Geometry check sheet. Reference: the model listing, model coordinates, mm. Give positions to 0.01 mm unless a question says otherwise; leave off trailing zeros. Order: outer loops, then holes, each group sorted by start corner. A loop starts at its lowest first (then second) coordinate and runs counter-clockwise, first axis right, second up.
from build123d import *

# Parameters (mm, degrees)
F0_R     = 10
F0_R_2   = 2.5
F1_DEPTH = 20
F2_DEPTH = 25


with BuildPart() as f1:
    # F0 (on Top) → F1 (new body)
    with BuildSketch(Plane.XY):
        with BuildLine():
            ThreePointArc((8.333333, -23.570226), (20.412415, -14.433757), (25, 0))
            ThreePointArc((25, 0), (20.412415, 14.433757), (8.333333, 23.570226))
            ThreePointArc((8.333333, 23.570226), (-25, 0), (8.333333, -23.570226))
        make_face()
        Circle(F0_R, mode=Mode.SUBTRACT)
        with BuildLine():
            ThreePointArc((8.333333, 23.570226), (20.412415, 14.433757), (25, 0))
            ThreePointArc((25, 0), (20.412415, -14.433757), (8.333333, -23.570226))
            Line((8.333333, -23.570226), (61.666667, -4.714045))
            ThreePointArc((61.666667, -4.714045), (55, 0), (61.666667, 4.714045))
            Line((61.666667, 4.714045), (8.333333, 23.570226))
        make_face()
        with BuildLine():
            ThreePointArc((65, 0), (64.082483, 2.886751), (61.666667, 4.714045))
            ThreePointArc((61.666667, 4.714045), (55, 0), (61.666667, -4.714045))
            ThreePointArc((61.666667, -4.714045), (64.082483, -2.886751), (65, 0))
        make_face()
        with Locations((60, 0)):
            Circle(F0_R_2, mode=Mode.SUBTRACT)
    extrude(amount=F1_DEPTH)

    # F0 (on Top) → F2 (join)
    with BuildSketch(Plane.XY):
        with BuildLine():
            ThreePointArc((8.333333, -23.570226), (20.412415, -14.433757), (25, 0))
            ThreePointArc((25, 0), (20.412415, 14.433757), (8.333333, 23.570226))
            ThreePointArc((8.333333, 23.570226), (-25, 0), (8.333333, -23.570226))
        make_face()
        Circle(F0_R, mode=Mode.SUBTRACT)
    extrude(amount=F2_DEPTH)


solid = f1.part
Item 1: Draft check along Y on faces 1 (the flat face through (0, -11, 25)), 2 (the cylindrical face through (62.31, -0.96, 9.86)), 3 (the flat face through (34.627, -14.274, 9.86)). Enter one of: released by +Y, released by -Y, zero draft, split by the parting line, or undercut.
Reported:
face 1: zero draft
face 2: undercut
face 3: released by -Y
Item 2: Sectioned sample at D-D (x = 60). Enter the section's corners in (y, z).
Reported:
outline: (-5.3, 0) - (-2.5, 0) - (-2.5, 20) - (-5.3, 20) - close; (2.5, 0) - (5.3, 0) - (5.3, 20) - (2.5, 20) - close
Item 3: Sectioned sample at B-B (x = 0). Enter the section's corners in (y, z), and give its area (3 significant figures).
Reported:
outline: (-25, 0) - (-10, 0) - (-10, 25) - (-25, 25) - close; (10, 0) - (25, 0) - (25, 25) - (10, 25) - close
area: 750 mm2
Item 4: Sectioned sample at A-A (z = 2.25). Enter the section's corners in (x, y), and give its area (3 significant figures).
Reported:
outline: (8.33, -23.57) - (61.67, -4.71) arc R5 ccw to (61.67, 4.71) - (8.33, 23.57) arc R25 ccw (long way) to start; hole circle Ø20 at (0, 0); hole circle Ø5 at (60, 0)
area: 2,590 mm2
Item 5: Sectioned sample at C-C (y = 9). Enter the section's corners in (x, z), and give its area (3 significant figures).
Reported:
outline: (-23.32, 0) - (-4.36, 0) - (-4.36, 25) - (-23.32, 25) - close; (4.36, 0) - (49.54, 0) - (49.54, 20) - (23.32, 20) - (23.32, 25) - (4.36, 25) - close
area: 1,470 mm2
Item 6: Gauge pin test, flat ends, axial feed: pin 1 (1 mm diameter, centred on y = 1.5, z = 7.5, fed in from +X); pin 2 (6 mm diameter, centred on x = -6.5, z = 17.5, fed in from +Y); pin 3 (10 mm diameter, centred on x = 14, z = 18, fed in from -Y). Record the tip position at first contact, or that the pin passes through.
Reported:
pin 1: stops at x = 64.9
pin 2: stops at y = 24.75
pin 3: stops at y = -23.33
Item 7: Scan lines: L1, parallel to Y at x = 0, z = 19.5; L2, parallel to Y at x = 60, z = 14.75; L3, parallel to X at y = 3.5, z = 14.5. Record each from-to range of solid material in increasing order.
Reported:
L1: y = -25 to -10, 10 to 25
L2: y = -5.3 to -2.5, 2.5 to 5.3
L3: x = -24.75 to -9.37, 9.37 to 63.57
